CAD build for the part. Positions are in the model's coordinates, mm. A direction names the side the tool comes from. Round coordinates to 2 decimals unless told otherwise and drop trailing zeros. Put each result on its own line as item: value. Start each with the question number.
1. 3-axis set-ups, long thin cutter, end or side, ignore diameter. For faces 4 (the cylindrical face through (272.16, 7.73, -271.76)), 5 (the flat face through (63.5, 8, -36)): which of +Z, -Z, +X, -X, +Y, -Y reach the whole face in a straight line?
2. Saw through at A-A on y = 7.5. State how many separate pieces and enclosed holes the cut face has, and give its area (3 significant figures).
3. Drill centre lines: line 1 (X direction, y = 13, z = -156); line 2 (Z direction, x = 65, y = 14); line 3 (Z direction, x = 142.5, y = 14). Where is each one in solid material? Low to high. Write a range as from..to.
4. Pull direction Z, two halves, no side cores. Call faces 1 (the cylindrical face through (139.86, 7.73, -82.55)), 2 (the flat face through (138, 15.24, -142)), 3 (the flat face through (138, 8, 0)): pulls with the +Z half, pulls with the -Z half, needs draft (parallel to the pull), parting line crosses it, or undercut.
5. Flat gauge pin, fed straight in: P1, Ø7.5, axis at x = 14, y = 9, coming from the +Z side. Where does the tip first touch, or does it go through?
from build123d import *

# Parameters (mm, degrees)
SKETCH1_W           = 279.4
SKETCH1_H           = 279.4
BOSS_EXTRUDE1_DEPTH = 15.24
FILLET1_R           = 25.4
SKETCH2_W           = 15.24
SKETCH2_H           = 31.75
CUT_EXTRUDE1_DEPTH  = 396.425059398
SKETCH3_W           = 15.24
SKETCH3_H           = 58.166
CUT_EXTRUDE2_DEPTH  = 396.425059398
SKETCH5_R           = 1.905
CUT_EXTRUDE4_DEPTH  = 396.425059398
CUT_EXTRUDE5_DEPTH  = 396.425059398


with BuildPart() as part:
    # Sketch1 → Boss-Extrude1 (new body)
    with BuildSketch(Plane(origin=(0, 0, 0), x_dir=(1, 0, 0), z_dir=(0, 1, 0))):
        with Locations((139.7, 139.7)):
            Rectangle(SKETCH1_W, SKETCH1_H)
    extrude(amount=BOSS_EXTRUDE1_DEPTH)

    # Fillet1
    fillet1_edges = [part.edges().sort_by_distance(p)[0] for p in [
        (0, 7.62, -279.4),
        (279.4, 7.62, -279.4),
        (279.4, 7.62, 0),
        (0, 7.62, 0),
    ]]
    fillet(fillet1_edges, radius=FILLET1_R)

    # Sketch2 → Cut-Extrude1 (cut, through all)
    with BuildSketch(Plane(origin=(0, 15.24, 0), x_dir=(1, 0, 0), z_dir=(0, 1, 0))):
        with Locations((71.12, 243.205)):
            Rectangle(SKETCH2_W, SKETCH2_H)
        with Locations((208.28, 243.205)):
            Rectangle(SKETCH2_W, SKETCH2_H)
        with Locations((71.12, 36.195)):
            Rectangle(SKETCH2_W, SKETCH2_H)
        with Locations((208.28, 36.195)):
            Rectangle(SKETCH2_W, SKETCH2_H)
    extrude(amount=-CUT_EXTRUDE1_DEPTH, mode=Mode.SUBTRACT)

    # Sketch3 → Cut-Extrude2 (cut, through all)
    with BuildSketch(Plane(origin=(0, 15.24, 0), x_dir=(1, 0, 0), z_dir=(0, 1, 0))):
        with Locations((13.97, 139.7)):
            Rectangle(SKETCH3_W, SKETCH3_H)
        with Locations((265.43, 139.7)):
            Rectangle(SKETCH3_W, SKETCH3_H)
        with Locations((54.61, 139.7)):
            Rectangle(SKETCH3_W, SKETCH3_H)
        with Locations((224.79, 139.7)):
            Rectangle(SKETCH3_W, SKETCH3_H)
    extrude(amount=-CUT_EXTRUDE2_DEPTH, mode=Mode.SUBTRACT)

    # Sketch5 → Cut-Extrude4 (cut, through all)
    with BuildSketch(Plane.XZ):
        with Locations(Location((115.062, -12.7, 0), (0, 0, 270))):
            Circle(SKETCH5_R)
        with Locations(Location((164.338, -12.7, 0), (0, 0, 270))):
            Circle(SKETCH5_R)
        with Locations(Location((164.338, -51.308, 0), (0, 0, 270))):
            Circle(SKETCH5_R)
        with Locations(Location((115.062, -51.308, 0), (0, 0, 270))):
            Circle(SKETCH5_R)
    extrude(amount=-CUT_EXTRUDE4_DEPTH, mode=Mode.SUBTRACT)

    # Sketch6 → Cut-Extrude5 (cut, through all)
    with BuildSketch(Plane(origin=(0, 15.24, 0), x_dir=(1, 0, 0), z_dir=(0, 1, 0))):
        with BuildLine():
            Line((83.70466448, 128.27), (86.299558054, 128.27))
            ThreePointArc((86.299558054, 128.27), (85.09, 139.7), (86.299558054, 151.13))
            Line((86.299558054, 151.13), (83.70466448, 151.13))
            ThreePointArc((83.70466448, 151.13), (82.55, 139.7), (83.70466448, 128.27))
        make_face()
        with BuildLine():
            Line((128.27, 193.100441946), (128.27, 195.69533552))
            ThreePointArc((128.27, 195.69533552), (139.7, 196.85), (151.13, 195.69533552))
            Line((151.13, 195.69533552), (151.13, 193.100441946))
            ThreePointArc((151.13, 193.100441946), (139.7, 194.31), (128.27, 193.100441946))
        make_face()
        with BuildLine():
            Line((193.100441946, 128.27), (195.69533552, 128.27))
            ThreePointArc((195.69533552, 128.27), (196.85, 139.7), (195.69533552, 151.13))
            Line((195.69533552, 151.13), (193.100441946, 151.13))
            ThreePointArc((193.100441946, 151.13), (194.31, 139.7), (193.100441946, 128.27))
        make_face()
        with BuildLine():
            Line((151.13, 86.299558054), (151.13, 83.70466448))
            ThreePointArc((151.13, 83.70466448), (139.7, 82.55), (128.27, 83.70466448))
            Line((128.27, 83.70466448), (128.27, 86.299558054))
            ThreePointArc((128.27, 86.299558054), (139.7, 85.09), (151.13, 86.299558054))
        make_face()
    extrude(amount=-CUT_EXTRUDE5_DEPTH, mode=Mode.SUBTRACT)


solid = part.part
Return value:
1. face 4: -Z, +X, +Y, -Y
1. face 5: +Y, -Y
2. separate pieces: 1
2. enclosed holes: 16
2. area: 71,700 mm^2
3. line 1: x = 0..6.35, 21.59..46.99, 62.23..217.17, 232.41..257.81, 273.05..279.4
3. line 2: z = -279.4..-259.08, -227.33..-52.07, -20.32..0
3. line 3: z = -279.4..-196.78, -194.24..-85.16, -82.62..0
4. face 1: undercut
4. face 2: needs draft
4. face 3: pulls with the +Z half
5. P1: stops at z = -1.18
